from build123d import *

# Parameters (mm, degrees)
F0_W     = 95
F0_H     = 66
F0_W_2   = 80
F0_H_2   = 58
F0_W_3   = 68.5
F0_H_3   = 53
F1_DEPTH = 0.1
F2_DEPTH = 4.5
F3_W     = 6
F3_H     = 52
F4_DEPTH = 2
F5_W     = 110
F5_H     = 80
F5_R     = 1.75
F5_W_2   = 95
F5_H_2   = 66
F5_W_3   = 68.5
F5_H_3   = 53
F6_DEPTH = 1


with BuildPart() as f1:
    # F0 (on Top) → F1 (new body)
    with BuildSketch(Plane.XY):
        with Locations((-0.5, 0)):
            Rectangle(F0_W, F0_H)
        Rectangle(F0_W_2, F0_H_2, mode=Mode.SUBTRACT)
        Rectangle(F0_W_2, F0_H_2)
        with Locations((3.25, 0)):
            Rectangle(F0_W_3, F0_H_3, mode=Mode.SUBTRACT)
    extrude(amount=F1_DEPTH)

    # F0 (on Top) → F2 (join)
    with BuildSketch(Plane.XY):
        with Locations((-0.5, 0)):
            Rectangle(F0_W, F0_H)
        Rectangle(F0_W_2, F0_H_2, mode=Mode.SUBTRACT)
    extrude(amount=F2_DEPTH)

    # F3 (on face) → F4 (cut)
    with BuildSketch(Plane.XY.offset(4.5)):
        with Locations((-45, 0)):
            Rectangle(F3_W, F3_H)
    extrude(amount=-F4_DEPTH, mode=Mode.SUBTRACT)

    # F5 (on face) → F6 (join)
    with BuildSketch(Plane(origin=(0, 0, 0), x_dir=(1, 0, 0), z_dir=(0, 0, -1))):
        with Locations((-0.5, 0)):
            Rectangle(F5_W, F5_H)
        with Locations((-51.25, -35.75)):
            Circle(F5_R, mode=Mode.SUBTRACT)
        with Locations((50.25, -35.75)):
            Circle(F5_R, mode=Mode.SUBTRACT)
        with Locations((-51.25, 35.75)):
            Circle(F5_R, mode=Mode.SUBTRACT)
        with Locations((-0.5, 0)):
            Rectangle(F5_W_2, F5_H_2, mode=Mode.SUBTRACT)
        with Locations((50.25, 35.75)):
            Circle(F5_R, mode=Mode.SUBTRACT)
        with Locations((-0.5, 0)):
            Rectangle(F5_W_2, F5_H_2)
        with Locations((3.25, 0)):
            Rectangle(F5_W_3, F5_H_3, mode=Mode.SUBTRACT)
    extrude(amount=F6_DEPTH)


solid = f1.part
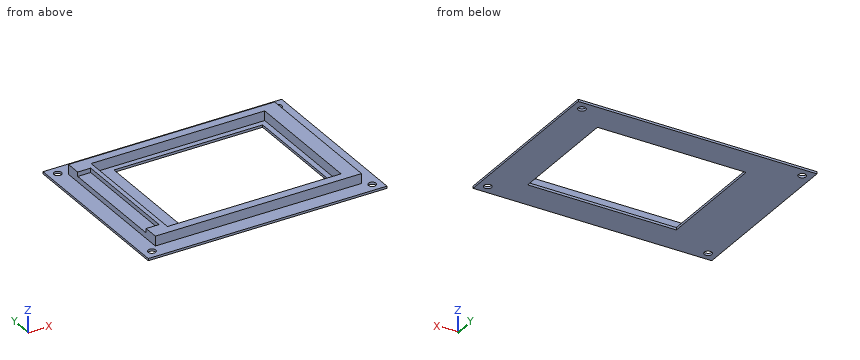
For this review, take the finished solid that the model builds, in its own axes (mm). Give positions to 0.01 mm unless a question says otherwise; leave off trailing zeros. Loops run counter-clockwise (first coordinate to the right, second up) from the corner with the lowest first, then second, coordinate; pieces in that order, holes last. Notation, with made-up numbers: (47.5, -1.5) -> (71.5, -1.5) arc R15 cw to (71.5, 15.5) -> close; hole circle Ø8 at (19.5, 29.25). An arc over 180 degrees is marked (long way). One line per question, with ' | ' between items.
1) Insertion check: pin 1 Ø4.5 at (x, y) = (-51.25, -35.75) entering from +Z; pin 2 Ø1.3 at (y, z) = (-11.5, 2) entering from -X; pin 3 Ø3 at (x, y) = (-51.25, 35.75) entering from +Z; pin 4 Ø5 at (x, y) = (-44, 9.5) entering from +Z. Each pin has a flat end and moves straight along its axis. Give the tip position at first contact, or say it passes through.
Resolved:
pin 1: stops at z = 0 | pin 2: stops at x = -48 | pin 3: passes through | pin 4: stops at z = 4.5
2) We need section D-D (y = -35.75). Write out the cut boundary in (x, z).
Resolved:
outline: (-55.5, -1) -> (-53, -1) -> (-53, 0) -> (-55.5, 0) -> close; (-49.5, -1) -> (48.5, -1) -> (48.5, 0) -> (-49.5, 0) -> close; (52, -1) -> (54.5, -1) -> (54.5, 0) -> (52, 0) -> close
3) We need section B-B (y = -19). Write out the cut boundary in (x, z), plus the area to 4 significant figures.
Resolved:
outline: (-55.5, -1) -> (-31, -1) -> (-31, 0.1) -> (-40, 0.1) -> (-40, 4.5) -> (-42, 4.5) -> (-42, 2.5) -> (-48, 2.5) -> (-48, 0) -> (-55.5, 0) -> close; (37.5, -1) -> (54.5, -1) -> (54.5, 0) -> (47, 0) -> (47, 4.5) -> (40, 4.5) -> (40, 0.1) -> (37.5, 0.1) -> close | area: 98.15 mm2
4) To check wall thickness, follow probe 1 along Y at (x, z) = (50.25, -0.25); probe 2 along X at (y, z) = (35.75, -0.7); probe 3 along X at (y, z) = (-6, 2.8). State the ranges of each line that lie inside material, in increasing order.
Resolved:
probe 1: y = -40 to -37.5, -34 to 34, 37.5 to 40 | probe 2: x = -55.5 to -53, -49.5 to 48.5, 52 to 54.5 | probe 3: x = -42 to -40, 40 to 47
5) We need section A-A (x = 26). Write out the cut boundary in (y, z), plus the area to 3 significant figures.
Resolved:
outline: (-40, -1) -> (-26.5, -1) -> (-26.5, 0.1) -> (-29, 0.1) -> (-29, 4.5) -> (-33, 4.5) -> (-33, 0) -> (-40, 0) -> close; (26.5, -1) -> (40, -1) -> (40, 0) -> (33, 0) -> (33, 4.5) -> (29, 4.5) -> (29, 0.1) -> (26.5, 0.1) -> close | area: 63.5 mm2
6) We need section C-C (x = 50.25). Write out the cut boundary in (y, z).
Resolved:
outline: (-40, -1) -> (-37.5, -1) -> (-37.5, 0) -> (-40, 0) -> close; (-34, -1) -> (34, -1) -> (34, 0) -> (-34, 0) -> close; (37.5, -1) -> (40, -1) -> (40, 0) -> (37.5, 0) -> close
